Autodesk Fusion 360 part; units mm, degrees
sketch "Top" plane through (0, 0, 0) normal (0, 0, 1) x (1, 0, 0)
  line L0 (-18, 0) -> (-138, 0)
  line L1 (-148, 10) -> (-148, 78)
  line L2 (-68, 158) -> (0, 158)
  line L3 (0, 158) -> (0, 58)
  line L4 (-138, 0) -> (-148, 10)
  line L5 (-18, 0) -> (-18, 58)
  line L6 (-18, 58) -> (0, 58)
  line L7 (-9, 158) -> (-9, 58) construction
  circle A0 centre (-9, 79) radius 3.5
  circle A1 centre (-9, 139) radius 3.5
  line L8 (-18, 49) -> (-148, 49) construction
  circle A2 centre (-43, 49) radius 3.5
  circle A3 centre (-118, 49) radius 3.5
  circle A4 centre (-43, 13) radius 6
  circle A5 centre (-68, 13) radius 3.5
  circle A6 centre (-68, 13) radius 7.5
  line L9 (-148, 78) -> (-68, 158)
  dimension "d4" = 158
  dimension "d5" = 10
  dimension "d6" = 10
  dimension "d7" = 58
  dimension "d8" = 18
  dimension "d9" = 148
  dimension "d11" = 9
  dimension "d12" = 7
  dimension "d13" = 7
  dimension "d14" = 21
  dimension "d15" = 60
  dimension "d16" = 49
  dimension "d17" = 7
  dimension "d18" = 7
  dimension "d19" = 25
  dimension "d20" = 75
  dimension "d21" = 12
  dimension "d22" = 13
  dimension "d23" = 7
  dimension "d24" = 15
  dimension "d25" = 25
  dimension "d26" = 25
  dimension "d27" = 68
  dimension "d28" = 68
extrude "Extrude1" add sketch "Top" along normal blind 13 contours A6
extrude "Extrude2" add sketch "Top" along normal blind 18 contours L0 L1 L2 L3 L4 L5 L6 L9
sketch "Side" plane through (-18, 0, 0) normal (1, 0, 0) x (0, 1, 0)
  line L0 (0, 0) -> (58, 0)
  line L1 (58, 0) -> (58, 18)
  line L2 (58, 18) -> (0, 18)
  line L3 (0, 18) -> (0, 0)
  line L4 (0, 0) -> (58, 0) construction
  line L5 (58, 0) -> (58, 18) construction
  line L6 (58, 18) -> (0, 18) construction
  line L7 (0, 18) -> (0, 0) construction
  line L8 (0, 9) -> (58, 9) construction
  circle A0 centre (13, 9) radius 3.5
  dimension "d33" = 7
  dimension "d34" = 13
extrude "Extrude3" cut sketch "Side" against normal blind 35 contours A0
Part model, mm, in its own coordinate system. A direction names the side the tool comes from. Give positions to 0.01 mm unless a question says otherwise; leave off trailing zeros. Loops run counter-clockwise (first coordinate to the right, second up) from the corner with the lowest first, then second, coordinate; pieces in that order, holes last. Notation, with made-up numbers: M 70,64 L 99,64 A17 cw 99,93 Z; hole C -36,70 d5. An arc over 180 degrees is marked long. Return JSON: item names as keys, results as strings.
1) Saw through at D-D, the plane y = 94. List the corners of the cut face in (x, z).
Calculated:
{"outline": "M -132,0 L 0,0 L 0,18 L -132,18 Z"}
2) Saw through at A-A, the plane x = -43. List the corners of the cut face in (y, z), then the cut area to 3 significant figures.
Calculated:
{"outline": "M 0,0 L 7,0 L 7,18 L 0,18 Z; M 19,0 L 45.5,0 L 45.5,18 L 19,18 Z; M 52.5,0 L 158,0 L 158,18 L 52.5,18 Z", "area": "2,500 mm2"}
3) Drill centre lines: line 1 (Y direction, x = -9, z = 9); line 2 (Y direction, x = -43, z = 8.75); line 3 (Y direction, x = -68, z = 6.5). Where is each one in solid material? Low to high.
Calculated:
{"line 1": "y = 58 to 75.5, 82.5 to 135.5, 142.5 to 158", "line 2": "y = 0 to 7, 19 to 45.5, 52.5 to 158", "line 3": "y = 0 to 9.5, 16.5 to 158"}
4) Flat gauge pins, fed straight in: pin 1 Ø3.5 at (y, z) = (12, 8.5) entering from +X; pin 2 Ø6 at (y, z) = (98, 14.5) entering from -X; pin 3 Ø4.5 at (x, y) = (-70.5, 15) entering from +Z. Where does each tip first touch, or does it go through?
Calculated:
{"pin 1": "stops at x = -53", "pin 2": "stops at x = -131", "pin 3": "stops at z = 13"}
5) Pull direction X, two halves, no side cores. Call faces 5 (the face through (-148, 44, 9)), 6 (the face through (-34, 158, 9)), 7 (the face through (-114.66, 47.95, 8.87)): released by +X, released by -X, zero draft, split by the parting line, or undercut.
Calculated:
{"face 5": "released by -X", "face 6": "zero draft", "face 7": "undercut"}
6) Saw through at B-B, the plane z = 9. List the corners of the cut face in (x, y).
Calculated:
{"outline": "M -148,10 L -138,0 L -18,0 L -18,9.5 L -38.13,9.5 A6 cw -47.87,9.5 L -53,9.5 L -53,16.5 L -47.87,16.5 A6 cw -38.13,16.5 L -18,16.5 L -18,58 L 0,58 L 0,158 L -68,158 L -148,78 Z; hole C -118,49 d7; hole C -68,13 d7; hole C -43,49 d7; hole C -9,79 d7; hole C -9,139 d7"}
7) 3-axis set-ups, long thin cutter, end or side, ignore diameter. For faces 1 (the face through (-69.8, 9.8, 13)), 2 (the face through (-27.923, 12.241, 5.583)), 3 (the face through (-9, 58, 9)), 4 (the face through (-109, 117, 9)): which of +Z, -Z, +X, -X, +Y, -Y reach the whole face in a straight line?
Calculated:
{"face 1": "+Z", "face 2": "+X", "face 3": "+Z, -Z, +X, -Y", "face 4": "+Z, -Z, -X, +Y"}
8) Saw through at C-C, the plane x = -118. List the corners of the cut face in (y, z).
Calculated:
{"outline": "M 0,0 L 45.5,0 L 45.5,18 L 0,18 Z; M 52.5,0 L 108,0 L 108,18 L 52.5,18 Z"}
